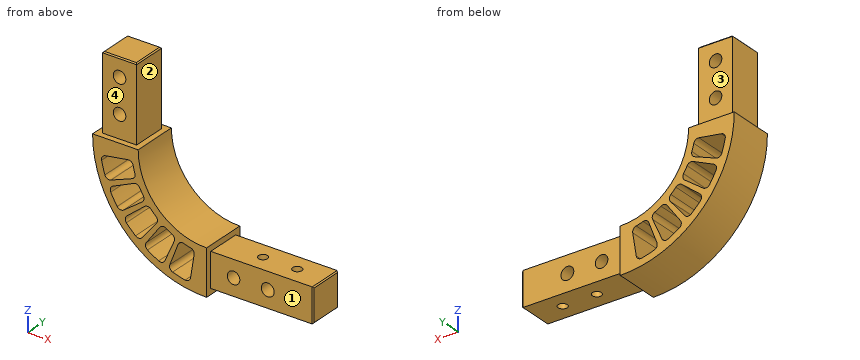
from build123d import *

# Parameters (mm, degrees)
BOSS_EXTRUDE1_DEPTH = 20
SKETCH2_W           = 15
SKETCH2_H           = 15
BOSS_EXTRUDE2_DEPTH = 33
SKETCH3_W           = 15
SKETCH3_H           = 15
BOSS_EXTRUDE3_DEPTH = 45
SKETCH4_R           = 2.75
SKETCH4_R_2         = 2.825
CUT_EXTRUDE1_DEPTH  = 73.844011422
CUT_EXTRUDE2_DEPTH  = 74.484692283
CHAMFER1_SIZE       = 0.5
SKETCH6_R           = 2
CUT_EXTRUDE3_DEPTH  = 20


with BuildPart() as part:
    # Sketch1 → Boss-Extrude1 (new body)
    with BuildSketch(Plane(origin=(0, 0, 0), x_dir=(1, 0, 0), z_dir=(0, 1, 0))):
        with BuildLine():
            Line((0, 50), (0, 30))
            ThreePointArc((0, 30), (-21.213203436, 21.213203436), (-30, 0))
            Line((-30, 0), (-50, 0))
            ThreePointArc((-50, 0), (-35.355339059, 35.355339059), (0, 50))
        make_face()
    extrude(amount=BOSS_EXTRUDE1_DEPTH)

    # Sketch2 → Boss-Extrude2 (add)
    with BuildSketch(Plane.XY):
        with Locations((-40, 10)):
            Rectangle(SKETCH2_W, SKETCH2_H)
    extrude(amount=BOSS_EXTRUDE2_DEPTH)

    # Sketch3 → Boss-Extrude3 (add)
    with BuildSketch(Plane(origin=(0, 0, 0), x_dir=(0, 0, -1), z_dir=(1, 0, 0))):
        with Locations((40, 10)):
            Rectangle(SKETCH3_W, SKETCH3_H)
    extrude(amount=BOSS_EXTRUDE3_DEPTH)

    # Sketch4 → Cut-Extrude1 (cut, through all)
    with BuildSketch(Plane(origin=(0, 17.5, 0), x_dir=(1, 0, 0), z_dir=(0, 1, 0))):
        with Locations(Location((10, 40, 0), (0, 0, 270))):
            Circle(SKETCH4_R)
        with Locations(Location((25, 40, 0), (0, 0, 270))):
            Circle(SKETCH4_R_2)
        with Locations(Location((-40, -10, 0), (0, 0, 270))):
            Circle(SKETCH4_R)
        with Locations(Location((-40, -25, 0), (0, 0, 270))):
            Circle(SKETCH4_R)
    extrude(amount=-CUT_EXTRUDE1_DEPTH, mode=Mode.SUBTRACT)

    # Sketch5 → Cut-Extrude2 (cut, through all)
    with BuildSketch(Plane(origin=(0, 20, 0), x_dir=(1, 0, 0), z_dir=(0, 1, 0))):
        with BuildLine():
            Line((-21.990223117, 27.155663999), (-28.291433976, 34.937011371))
            ThreePointArc((-28.291433976, 34.937011371), (-29.68093252, 35.671569812), (-31.172202606, 35.17518706))
            ThreePointArc((-31.172202606, 35.17518706), (-33.234018716, 33.234018716), (-35.17518706, 31.172202606))
            ThreePointArc((-35.17518706, 31.172202606), (-35.671569812, 29.68093252), (-34.937011371, 28.291433976))
            Line((-34.937011371, 28.291433976), (-27.155663999, 21.990223117))
            ThreePointArc((-27.155663999, 21.990223117), (-25.744904759, 21.550308438), (-24.417193319, 22.199114181))
            ThreePointArc((-24.417193319, 22.199114181), (-23.334523779, 23.334523779), (-22.199114181, 24.417193319))
            ThreePointArc((-22.199114181, 24.417193319), (-21.550308438, 25.744904759), (-21.990223117, 27.155663999))
        make_face()
        with BuildLine():
            Line((-20.538868638, 28.26932746), (-26.424199651, 36.369790662))
            ThreePointArc((-26.424199651, 36.369790662), (-26.774099933, 37.902060905), (-25.908661914, 39.214043885))
            ThreePointArc((-25.908661914, 39.214043885), (-23.5, 40.703193978), (-21.006027233, 42.044581338))
            ThreePointArc((-21.006027233, 42.044581338), (-19.437097633, 42.138081158), (-18.285062818, 41.068923503))
            Line((-18.285062818, 41.068923503), (-14.21252141, 31.921845736))
            ThreePointArc((-14.21252141, 31.921845736), (-14.152727818, 30.445298653), (-15.123063049, 29.330751167))
            ThreePointArc((-15.123063049, 29.330751167), (-16.5, 28.578838325), (-17.839644098, 27.762332367))
            ThreePointArc((-17.839644098, 27.762332367), (-19.290038151, 27.47927115), (-20.538868638, 28.26932746))
        make_face()
        with BuildLine():
            Line((-12.522383321, 32.621923854), (-16.110622392, 41.969606219))
            ThreePointArc((-16.110622392, 41.969606219), (-16.05201939, 43.540226476), (-14.876504274, 44.583512878))
            ThreePointArc((-14.876504274, 44.583512878), (-12.16449512, 45.398513836), (-9.408325818, 46.04870688))
            ThreePointArc((-9.408325818, 46.04870688), (-7.868656664, 45.73295191), (-7.032594847, 44.402056368))
            Line((-7.032594847, 44.402056368), (-5.466259855, 34.512606439))
            ThreePointArc((-5.466259855, 34.512606439), (-5.790662187, 33.070895758), (-7.016400163, 32.245466794))
            ThreePointArc((-7.016400163, 32.245466794), (-8.541028488, 31.875552268), (-10.046352613, 31.433593482))
            ThreePointArc((-10.046352613, 31.433593482), (-11.52058732, 31.535566946), (-12.522383321, 32.621923854))
        make_face()
        with BuildLine():
            Line((-31.921845736, 14.21252141), (-41.068923503, 18.285062818))
            ThreePointArc((-41.068923503, 18.285062818), (-42.138081158, 19.437097633), (-42.044581338, 21.006027233))
            ThreePointArc((-42.044581338, 21.006027233), (-40.703193978, 23.5), (-39.214043885, 25.908661914))
            ThreePointArc((-39.214043885, 25.908661914), (-37.902060905, 26.774099933), (-36.369790662, 26.424199651))
            Line((-36.369790662, 26.424199651), (-28.26932746, 20.538868638))
            ThreePointArc((-28.26932746, 20.538868638), (-27.47927115, 19.290038151), (-27.762332367, 17.839644098))
            ThreePointArc((-27.762332367, 17.839644098), (-28.578838325, 16.5), (-29.330751167, 15.123063049))
            ThreePointArc((-29.330751167, 15.123063049), (-30.445298653, 14.152727818), (-31.921845736, 14.21252141))
        make_face()
        with BuildLine():
            Line((-34.512606439, 5.466259855), (-44.402056368, 7.032594847))
            ThreePointArc((-44.402056368, 7.032594847), (-45.73295191, 7.868656664), (-46.04870688, 9.408325818))
            ThreePointArc((-46.04870688, 9.408325818), (-45.398513836, 12.16449512), (-44.583512878, 14.876504274))
            ThreePointArc((-44.583512878, 14.876504274), (-43.540226476, 16.05201939), (-41.969606219, 16.110622392))
            Line((-41.969606219, 16.110622392), (-32.621923854, 12.522383321))
            ThreePointArc((-32.621923854, 12.522383321), (-31.535566946, 11.52058732), (-31.433593482, 10.046352613))
            ThreePointArc((-31.433593482, 10.046352613), (-31.875552268, 8.541028488), (-32.245466794, 7.016400163))
            ThreePointArc((-32.245466794, 7.016400163), (-33.070895758, 5.790662187), (-34.512606439, 5.466259855))
        make_face()
    extrude(amount=-CUT_EXTRUDE2_DEPTH, mode=Mode.SUBTRACT)

    # Chamfer1
    chamfer1_edges = [part.edges().sort_by_distance(p)[0] for p in [
        (-32.5, 10, 33),
        (-40, 17.5, 33),
        (-47.5, 10, 33),
        (-40, 2.5, 33),
        (45, 10, -47.5),
        (45, 17.5, -40),
        (45, 10, -32.5),
        (45, 2.5, -40),
    ]]
    chamfer(chamfer1_edges, length=CHAMFER1_SIZE)

    # Sketch6 → Cut-Extrude3 (cut)
    with BuildSketch(Plane(origin=(0, 0, -47.5), x_dir=(-1, 0, 0), z_dir=(0, 0, -1))):
        with Locations((-17.5, 10)):
            Circle(SKETCH6_R)
        with Locations((-32.5, 10)):
            Circle(SKETCH6_R)
    extrude(amount=-CUT_EXTRUDE3_DEPTH, mode=Mode.SUBTRACT)


solid = part.part
Build history of the part. All positions in model axes, mm. Face numbers are marked on the shaded views. A direction names the side the tool comes from. Give positions to 0.01 mm unless a question says otherwise; leave off trailing zeros. Order: outer loops, then holes, each group sorted by start corner. A loop starts at its lowest first (then second) coordinate and runs counter-clockwise, first axis right, second up. Notation, with made-up numbers: M -34.5,22 L 9.5,22 A16 ccw 9.5,53 Z; hole C 77,76.25 d3. An arc over 180 degrees is marked long. Put each result on its own line as item: value.
Item 1: Which spindle directions (+Z, -Z, +X, -X, +Y, -Y) get a long thin tool onto all of the face, cutting with end or side? Do the marked faces 1, 2, 3 and 4. Say none if no direction does.
Results are:
face 1: +Z, -Z, +X, -Y
face 2: +Z, +X, +Y, -Y
face 3: +Z, +X, -X, +Y
face 4: +Z, +X, -X, -Y
Item 2: Cut at A-A on x = 25. Write the cut outline in (y, z) (3 decimals).
Results are:
outline: M 2.5,-47.5 L 17.5,-47.5 L 17.5,-42.825 L 2.5,-42.825 Z; M 2.5,-37.175 L 17.5,-37.175 L 17.5,-32.5 L 2.5,-32.5 Z
Item 3: Cut at B-B on z = 25. Write the cut outline in (x, y).
Results are:
outline: M -47.5,2.5 L -42.75,2.5 L -42.75,17.5 L -47.5,17.5 Z; M -37.25,2.5 L -32.5,2.5 L -32.5,17.5 L -37.25,17.5 Z
Item 4: Drop flat-ended pins along their axis: pin 1 Ø1.5 at (y, z) = (16.5, 13) entering from +X; pin 2 Ø7.5 at (x, z) = (25, -40) entering from -Y; pin 3 Ø6 at (x, y) = (8, 17) entering from -Z; pin 4 Ø3.5 at (x, y) = (17.5, 10) entering from -Z. Give the stop position or say it passes through.
Results are:
pin 1: x = -32.5
pin 2: y = 2.5
pin 3: z = -47.5
pin 4: through
Item 5: Wall check: probe 1 along X at (y, z) = (14.25, 10); probe 2 along X at (y, z) = (18.25, -40.5); probe 3 along X at (y, z) = (5, -22). Give the ranges that are in metal, low to high.
Results are:
probe 1: -47.5 to -42.75, -37.25 to -32.5
probe 2: -29.32 to -23.85, -18.03 to -15.55, -6.41 to 0
probe 3: -44.9 to -41.53, -30.28 to -27.17, -24.63 to -20.4
